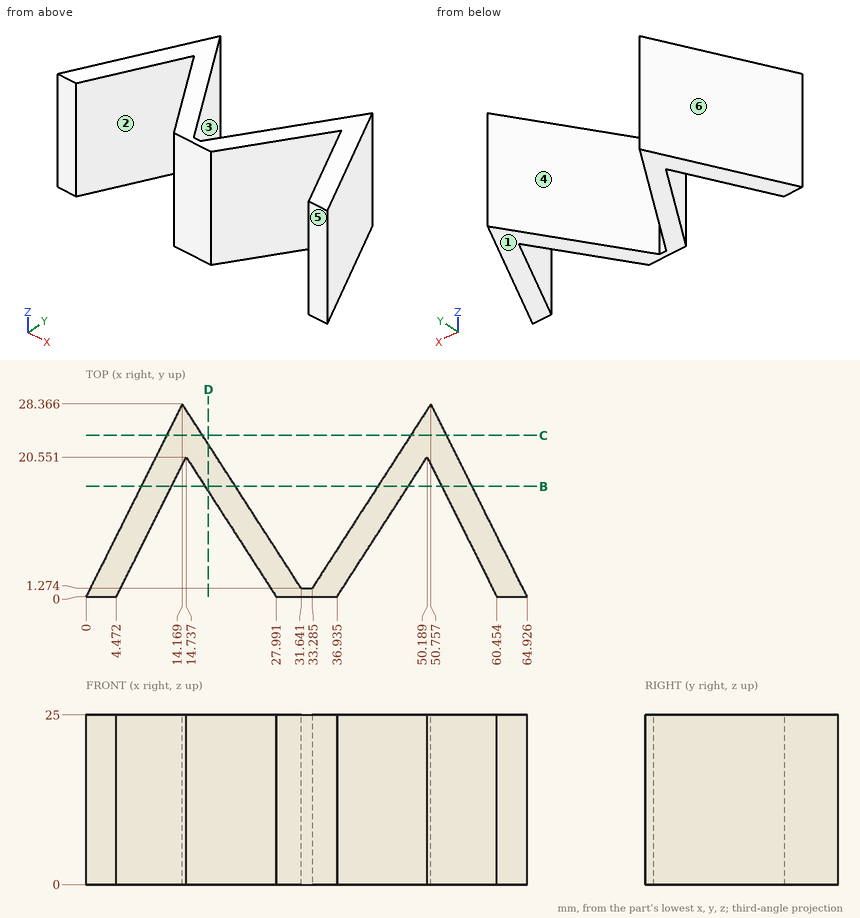
Design review of the part shown in the three views and the two pictorial views. Dimensions are in mm from the part's minimum x, y and z. A direction names the side the tool comes from. Coordinates: 2 decimals unless noted, no trailing zeros. Order: outer loops, then holes, each group sorted by start corner. A loop starts at its lowest first (then second) coordinate and runs counter-clockwise, first axis right, second up.
1) Take a section at D-D, the plane x = 18. Give the boundary of the cut face in (y, z) (1 decimal).
2) Wall thickness on line 1 along X through (y, z) = (10.5, 17.5) (1 decimal); line 2 along X through (y, z) = (3, 10.25) (1 decimal); line 3 along X through (y, z) = (23.5, 1.75) (1 decimal): over which ranges is each line inside the solid? List them lowest first.
3) Clearance check with flat-ended pins moving along their axes: pin 1 (12 mm diameter, centred on y = 12.5, z = 11, fed in from -X); pin 2 (5 mm diameter, centred on x = 25, z = 20.5, fed in from +Y); pin 3 (1 mm diameter, centred on y = 15, z = 8.5, fed in from -X); pin 4 (1 mm diameter, centred on x = 36.5, y = 7.5, fed in from +Z). State where each tip first meets the part, or that it passes through.
4) For the marked faces 1, 2 and 3, list the 3-axis set-ups (+Z, -Z, +X, -X, +Y, -Y) from which the entire face can be reached by the end or side of a thin tool; tool diameter is ignored.
5) Mouldability with a two-part tool opening along X and no side actions: class the marked faces 4, 5 and 6 as +X half, -X half, draft (parallel to the pull), parting line (faces both ways), or undercut.
6) Take a section at B-B, the plane y = 16.25. Give the boundary of the cut face in (x, z) (1 decimal).
7) Take a section at C-C, the plane y = 23.75. Give the boundary of the cut face in (x, z) (1 decimal), and give its area (3 significant figures).
Returned:
1. outline: (15.5, 0) - (22.4, 0) - (22.4, 25) - (15.5, 25) - close
2. line 1: x = 5.2 to 9.7, 21.2 to 25.7, 39.2 to 43.7, 55.2 to 59.7
2. line 2: x = 1.5 to 6, 26.1 to 30.5, 34.4 to 38.9, 59 to 63.4
2. line 3: x = 11.7 to 17.3, 47.6 to 53.2
3. pin 1: stops at x = 3.25
3. pin 2: stops at y = 15.45
3. pin 3: stops at x = 7.24
3. pin 4: passes through
4. face 1: -Z, +X, -X, +Y, -Y
4. face 2: +Z, -Z, -Y
4. face 3: +Z, -Z, +Y
5. face 4: undercut
5. face 5: draft
5. face 6: -X half
6. outline: (8.1, 0) - (12.6, 0) - (12.6, 25) - (8.1, 25) - close; (17.5, 0) - (22, 0) - (22, 25) - (17.5, 25) - close; (42.9, 0) - (47.4, 0) - (47.4, 25) - (42.9, 25) - close; (52.3, 0) - (56.8, 0) - (56.8, 25) - (52.3, 25) - close
7. outline: (11.9, 0) - (17.1, 0) - (17.1, 25) - (11.9, 25) - close; (47.8, 0) - (53.1, 0) - (53.1, 25) - (47.8, 25) - close
7. area: 264 mm2
